```python
from build123d import *
from OCP.BRepFilletAPI import BRepFilletAPI_MakeChamfer

# Parameters (mm, degrees)
EXTRUDE_1_DEPTH = 3.9
EXTRUDE_2_DEPTH = 35.65
CHAMFER_1_SIZE  = 8
CHAMFER_1_SIZE2 = 3.35
CHAMFER_2_SIZE  = 8
EXTRUDE_3_DEPTH = 2.4


with BuildPart() as part:
    # 草图1 → 凸台-拉伸1 (new, symmetric)
    with BuildSketch(Plane.XY):
        Polygon((-37, 0), (0, 0), (0, 37), (-7.5, 37), (-7.5, 7.5), (-37, 7.5), align=None)
    extrude(amount=EXTRUDE_1_DEPTH, both=True)

    # 草图3 → 凸台-拉伸2 (add)
    with BuildSketch(Plane.ZY.offset(37)):
        Polygon((-3.9, 0), (-7.25, 4.174374383), (-7.25, 6), (-3.9, 6), align=None)
        Polygon((3.9, 6), (3.9, 0), (7.25, 4.174374383), (7.25, 6), align=None)
    extrude(amount=-EXTRUDE_2_DEPTH)

    # 倒角1: one chamfer whose edges measure the first distance from different faces: ONE call of the kernel's chamfer builder (chamfer() names one face for all edges)
    chamfer_1_edges_1 = [part.edges().sort_by_distance(p)[0] for p in [
        (-37, 5.087187192, -7.25),
    ]]
    chamfer_1_side_1 = [part.faces().sort_by_distance(p)[0] for p in [
        (-19.175, 5.087187192, -7.25),
    ]]
    chamfer_1_edges_2 = [part.edges().sort_by_distance(p)[0] for p in [
        (-37, 5.087187192, 7.25),
    ]]
    chamfer_1_side_2 = [part.faces().sort_by_distance(p)[0] for p in [
        (-19.175, 5.087187192, 7.25),
    ]]
    chamfer_1 = BRepFilletAPI_MakeChamfer(part.part.solid().wrapped)
    for e in chamfer_1_edges_1:
        chamfer_1.Add(CHAMFER_1_SIZE, CHAMFER_1_SIZE2, e.wrapped, chamfer_1_side_1[0].wrapped)  # the first distance lies on this face
    for e in chamfer_1_edges_2:
        chamfer_1.Add(CHAMFER_1_SIZE, CHAMFER_1_SIZE2, e.wrapped, chamfer_1_side_2[0].wrapped)  # the first distance lies on this face
    add(Compound.cast(chamfer_1.Shape()), mode=Mode.REPLACE)

    # 倒角2
    # the kernel refuses this chamfer: 8 mm, written as the material it takes off along each edge
    with BuildSketch(Plane(origin=(-1.35, -16.39908952, 7.25), x_dir=(-0.9996219169112968, 0, 0.027495876610586382), z_dir=(0, 1, 0))) as chamfer_2_piece_1_section:
        Polygon((CHAMFER_2_SIZE * 0.999621916911, -CHAMFER_2_SIZE * 0.0274958766106), (-CHAMFER_2_SIZE * 0.0274958766106, -CHAMFER_2_SIZE * 0.999621916911), (0, 0), align=None)
    chamfer_2_piece_1 = extrude(amount=42.972553424, mode=Mode.PRIVATE)
    chamfer_2_piece_1 = split(chamfer_2_piece_1, bisect_by=Plane(origin=(-4.629145345, 5.087187192, 3.9), z_dir=(0, 0, 1)), keep=Keep.TOP, mode=Mode.PRIVATE)
    add(chamfer_2_piece_1, mode=Mode.SUBTRACT)
    with BuildSketch(Plane(origin=(-1.35, -16.39908952, -7.25), x_dir=(-0.9996219169112968, 0, -0.027495876610586382), z_dir=(0, 1, 0))) as chamfer_2_piece_2_section:
        Polygon((CHAMFER_2_SIZE * 0.999621916911, CHAMFER_2_SIZE * 0.0274958766106), (-CHAMFER_2_SIZE * 0.0274958766106, CHAMFER_2_SIZE * 0.999621916911), (0, 0), align=None)
    chamfer_2_piece_2 = extrude(amount=42.972553424, mode=Mode.PRIVATE)
    chamfer_2_piece_2 = split(chamfer_2_piece_2, bisect_by=Plane(origin=(-4.629145345, 5.087187192, -3.9), z_dir=(0, 0, -1)), keep=Keep.TOP, mode=Mode.PRIVATE)
    add(chamfer_2_piece_2, mode=Mode.SUBTRACT)

    # 草图4 → 凸台-拉伸3 (add, symmetric)
    with BuildSketch(Plane.ZY.offset(3.75)):
        with BuildLine():
            Line((-3.9, 37), (-4.25, 37))
            ThreePointArc((-4.25, 37), (-6.371320344, 36.121320344), (-7.25, 34))
            Line((-7.25, 34), (-7.25, 16))
            ThreePointArc((-7.25, 16), (-6.371320344, 13.878679656), (-4.25, 13))
            Line((-4.25, 13), (-3.9, 13))
            Line((-3.9, 13), (-3.9, 37))
        make_face()
        with BuildLine():
            Line((3.9, 37), (3.9, 13))
            Line((3.9, 13), (4.25, 13))
            ThreePointArc((4.25, 13), (6.371320344, 13.878679656), (7.25, 16))
            Line((7.25, 16), (7.25, 34))
            ThreePointArc((7.25, 34), (6.371320344, 36.121320344), (4.25, 37))
            Line((4.25, 37), (3.9, 37))
        make_face()
    extrude(amount=EXTRUDE_3_DEPTH, both=True)

    # 草图6 → M6 螺纹孔1 (revolve, cut)
    with BuildSketch(Plane(origin=(-24.5, 7.5, 0), x_dir=(0, 0, 1), z_dir=(1, 0, 0))):
        Polygon((0, 0), (0, 29.502151548), (2.5, 28), (2.5, 0), align=None)
    hole_wizard_m6_1 = revolve(axis=Axis((-24.5, 13.85, 0), (0, -1, 0)), mode=Mode.SUBTRACT)

    # 镜向1: M6 螺纹孔1 across plane
    add(hole_wizard_m6_1.mirror(Plane(origin=(0, 0, 0), x_dir=(0, 0, 1), z_dir=(-0.7071067811865477, -0.7071067811865475, 0))), mode=Mode.SUBTRACT)


solid = part.part
```
Here's how the part is built. I have some questions about the finished solid (model axes, mm). A direction names the side the tool comes from. Coordinates: 2 decimals unless noted, no trailing zeros. Order: outer loops, then holes, each group sorted by start corner. A loop starts at its lowest first (then second) coordinate and runs counter-clockwise, first axis right, second up. Notation, with made-up numbers: M 7.5,35.25 L 43.5,35.25 A21 ccw 43.5,39.25 Z; hole C 50,-34.75 d11. An arc over 180 degrees is marked long. Answer as a JSON object with one key per item and string values. Group by question number.
(1) Suppose I cut it at D-D, the plane y = 5.5. Please give me the cut outline in (x, z), then the cut area to 3 significant figures.
(2) I need wall thicknesses on probe 1 along X at (y, z) = (5, 0); probe 2 along Y at (x, z) = (-4.75, 0); probe 3 along X at (y, z) = (32, 1). Which ranges of each line are inside material? Lowest first, please.
(3) If we mould it in two halves opening along X, with no side actions, what happens to faces 4 (the face through (-27, 4, 0)), 5 (the face through (-3.72, 36.14, -6.35)), 6 (the face through (-7.3, 3.6, 5.2))? For each: released by +X, released by -X, zero draft, split by the parting line, or undercut.
(4) Suppose I cut it at A-A, the plane x = -24.5. Please give me the cut outline in (y, z).
(5) Which directions (+Z, -Z, +X, -X, +Y, -Y) give clear straight access to the entire face, cutting with the end or side of a thin tool? Please do faces 1 (the face through (-7.5, 22, 2)), 2 (the face through (-1.35, 25, -6)), 3 (the face through (-22, 6, 6)).
(6) For pin 1 (6 mm diameter, centred on x = -23, z = 2, fed in from +Y); pin 2 (1 mm diameter, centred on x = -17.5, z = -5.5, fed in from +Y); pin 3 (2.5 mm diameter, centred on y = 21, z = -5.5, fed in from +X), each with a flat end and sliding along its axis, tell me the tip position at first contact or that it passes through.
(7) Suppose I cut it at B-B, the plane z = 0. Please give me the cut outline in (x, y), then the cut area to 3 significant figures.
(8) Suppose I cut it at C-C, the plane y = 24.5. Please give me the cut outline in (x, z).
Values found:
{
 "1": {"outline": "M -37,-3.9 L -29,-7.25 L -9.35,-7.25 L -6,-3.9 L 0,-3.9 L 0,3.9 L -6,3.9 L -9.35,7.25 L -29,7.25 L -37,3.9 Z; hole C -24.5,0 d5", "area": "439 mm^2"},
 "2": {"probe 1": "x = -37 to -27, -22 to 0", "probe 2": "y = 0 to 22, 27 to 37", "probe 3": "x = -7.5 to 0"},
 "3": {"face 4": "undercut", "face 5": "zero draft", "face 6": "released by +X"},
 "4": {"outline": "M 0,-3.9 L 4.17,-7.25 L 6,-7.25 L 6,-3.9 L 7.5,-3.9 L 7.5,-2.5 L 0,-2.5 Z; M 0,2.5 L 7.5,2.5 L 7.5,3.9 L 6,3.9 L 6,7.25 L 4.17,7.25 L 0,3.9 Z"},
 "5": {"face 1": "+Z, -Z, -X, +Y", "face 2": "-Z, +X, +Y, -Y", "face 3": "+Z, +X, -X, +Y"},
 "6": {"pin 1": "stops at y = 7.5", "pin 2": "stops at y = 6", "pin 3": "stops at x = -1.35"},
 "7": {"outline": "M -37,0 L -27,0 L -27,7.5 L -37,7.5 Z; M -22,0 L 0,0 L 0,22 L -7.5,22 L -7.5,7.5 L -22,7.5 Z; M -7.5,27 L 0,27 L 0,37 L -7.5,37 Z", "area": "424 mm^2"},
 "8": {"outline": "M -7.5,-3.9 L -6.15,-3.9 L -6.15,-7.25 L -1.35,-7.25 L -1.35,-3.9 L 0,-3.9 L 0,-2.5 L -7.5,-2.5 Z; M -7.5,2.5 L 0,2.5 L 0,3.9 L -1.35,3.9 L -1.35,7.25 L -6.15,7.25 L -6.15,3.9 L -7.5,3.9 Z"}
}
